from build123d import *

# Parameters (mm, degrees)
SKETCH1_W           = 71
SKETCH1_H           = 81
SKETCH1_R           = 1.5
BOSS_EXTRUDE1_DEPTH = 5
FILLET1_R           = 8


with BuildPart() as part:
    # Sketch1 → Boss-Extrude1 (new body)
    with BuildSketch(Plane(origin=(0, 0, 0), x_dir=(0, 0, -1), z_dir=(1, 0, 0))):
        with Locations((35.5, 40.5)):
            Rectangle(SKETCH1_W, SKETCH1_H)
        with Locations((6, 75)):
            Circle(SKETCH1_R, mode=Mode.SUBTRACT)
        with Locations((65, 75)):
            Circle(SKETCH1_R, mode=Mode.SUBTRACT)
        with Locations((6, 16)):
            Circle(SKETCH1_R, mode=Mode.SUBTRACT)
        with Locations((65, 16)):
            Circle(SKETCH1_R, mode=Mode.SUBTRACT)
    extrude(amount=BOSS_EXTRUDE1_DEPTH)

    # Fillet1
    fillet1_edges = [part.edges().sort_by_distance(p)[0] for p in [
        (2.5, 81, 0),
        (2.5, 81, -71),
    ]]
    fillet(fillet1_edges, radius=FILLET1_R)


solid = part.part
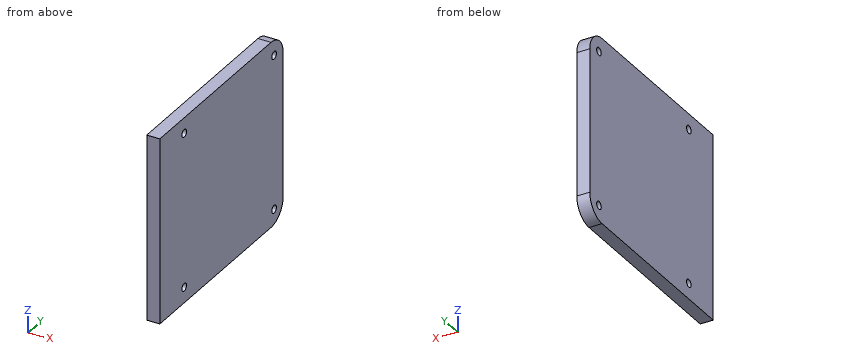
Work out the finished part from the listing and answer in its coordinate system (mm). Coordinates: 2 decimals unless noted, no trailing zeros. Loops run counter-clockwise (first coordinate to the right, second up) from the corner with the lowest first, then second, coordinate; pieces in that order, holes last. Notation, with made-up numbers: M 65,-13.5 L 98,-13.5 A24 cw 98,18.5 Z; hole C 26.5,66.5 d10. An arc over 180 degrees is marked long. Answer in a Markdown table with one row per item. Add a question column.
1. Find section A-A, the plane y = 16. Write down the section's boundary in (x, z), then the cut area to 3 significant figures.
2. Find section B-B, the plane z = -6. Write down the section's boundary in (x, y), then the cut area to 3 significant figures.
3. Flat-ended cylindrical pins translate along their axes: P1, Ø4, axis at y = 75, z = -6, coming from the +X side; P2, Ø2.5, axis at y = 75, z = -65, coming from the -X side. Find the tip coordinate at first contact, or state that the pin passes through.
4. Consider L1, parallel to Y at x = 2.2, z = -64; L2, parallel to Z at x = 3.7, y = 75; L3, parallel to Y at x = 0.8, z = -66. Determine where each line is inside the solid, lowest interval first.
Reported:
| question | item | result |
|---|---|---|
| 1 | outline | M 0,-71 L 5,-71 L 5,-66.5 L 0,-66.5 Z; M 0,-63.5 L 5,-63.5 L 5,-7.5 L 0,-7.5 Z; M 0,-4.5 L 5,-4.5 L 5,0 L 0,0 Z |
| 1 | area | 325 mm^2 |
| 2 | outline | M 0,0 L 5,0 L 5,14.5 L 0,14.5 Z; M 0,17.5 L 5,17.5 L 5,73.5 L 0,73.5 Z; M 0,76.5 L 5,76.5 L 5,80.75 L 0,80.75 Z |
| 2 | area | 374 mm^2 |
| 3 | P1 | stops at x = 5 |
| 3 | P2 | passes through |
| 4 | L1 | y = 0 to 14.88, 17.12 to 73.88, 76.12 to 80.94 |
| 4 | L2 | z = -70.75 to -66.5, -63.5 to -7.5, -4.5 to -0.25 |
| 4 | L3 | y = 0 to 14.88, 17.12 to 73.88, 76.12 to 80.42 |
